Source: CAD feature listing. Evaluate the final solid. Frame: model axes, mm. A direction names the side the tool comes from. Round coordinates to 2 decimals unless told otherwise and drop trailing zeros. Order: outer loops, then holes, each group sorted by start corner. A loop starts at its lowest first (then second) coordinate and runs counter-clockwise, first axis right, second up. Notation, with made-up numbers: (67, 57) -> (100, 57) arc R18 cw to (100, 61) -> close; hole circle Ø3 at (52.25, 75.25). An arc over 180 degrees is marked (long way). One line per item, written item: value. Start each with the question number.
1) Section B-B (z = -34). Return the cut outline in (x, y) (1 decimal), and give its area (3 significant figures).
2) Mould query, pull axis X, two halves, no side actions, for faces 4 (the face through (12.7, 3, 28)), 5 (the face through (79, 3, -40.005)), 6 (the face through (16.43, 2.8, -14.05)), 7 (the face through (15.875, 3, 0)). Classes: pulls with the +X half, pulls with the -X half, needs draft (parallel to the pull), parting line crosses it, or undercut.
3) Section C-C (x = 33). Return the cut outline in (y, z) (3 decimals), and give its area (3 significant figures).
4) Section D-D (z = 5). Return the cut outline in (x, y) (1 decimal), and give its area (3 significant figures).
5) Pin query (flat end, axial travel): P1, Ø1.7, axis at y = 4, z = 11.5, coming from the +X side; P2, Ø3, axis at x = -7, y = 2, coming from the +Z side; P3, Ø1.6, axis at y = 3, z = -15, coming from the +X side. Return the tip coordinate at first contact, or that it passes through.
6) Section A-A (x = 0). Return the cut outline in (y, z) (3 decimals), and give its area (3 significant figures).
7) Reachability of faces 1 (the face through (74.295, 3, -36)), 2 (the face through (55.116, 2.885, -8.868)), 3 (the face through (28.499, 3, -32)) from +Z, -Z, +X, -X, +Y, -Y: full face, straight path, thin tool, end or side. Return the list, or none.
8) Ray query, L1, parallel to X at y = 5.05, z = -33 (1 decimal); L2, parallel to Z at x = 35, y = 3.15 (3 decimals); L3, parallel to X at y = 1.2, z = -26.67. Return the intervals inside material, ascending.
```python
from build123d import *

# Parameters (mm, degrees)
SKETCH1_W                   = 33.3375
SKETCH1_H                   = 41.1861
BOSS_EXTRUDE1_DEPTH         = 5.6896
FILLET1_R                   = 12.7
FILLET2_R                   = 6.35
CUT_EXTRUDE3_REACH          = 7.69
SKETCH11_R                  = 6.35
SKETCH8_W                   = 12.7
SKETCH8_H                   = 3.175
CUT_EXTRUDE2_DEPTH          = 5.6896
F_4_CLEARANCE_HOLE3_D       = 2.9464
F_4_CLEARANCE_HOLE3_DEPTH   = 5.6906
CIRPATTERN1_COUNT           = 4
FILLET3_R                   = 12.7
F_4_CLEARANCE_HOLE4_D       = 2.9464
TAP_DRILL_FOR_4_HELICOIL1_D = 3.9878
FILLET4_R                   = 6.35


with BuildPart() as part:
    # Sketch1 → Boss-Extrude1 (new body)
    with BuildSketch(Plane(origin=(0, 0, 0), x_dir=(1, 0, 0), z_dir=(0, 1, 0))):
        with BuildLine():
            Line((28.4988, 40.005), (28.4988, 24.13))
            Line((28.4988, 24.13), (0, 24.13))
            Line((0, 24.13), (-24.13, 24.13))
            Line((-24.13, 24.13), (-24.13, 0))
            Line((-24.13, 0), (-24.13, -24.13))
            Line((-24.13, -24.13), (0, -24.13))
            Line((0, -24.13), (12.7, -24.13))
            Line((12.7, -24.13), (12.7, -38.1))
            Line((12.7, -38.1), (71.8185, -38.1))
            Line((71.8185, -38.1), (71.8185, 7.9375))
            Line((71.8185, 7.9375), (84.5185, 20.6375))
            Line((84.5185, 20.6375), (84.5185, 40.005))
            Line((84.5185, 40.005), (74.295, 40.005))
            Line((74.295, 40.005), (74.295, 31.75))
            ThreePointArc((74.295, 31.75), (66.675, 24.13), (59.055, 31.75))
            Line((59.055, 31.75), (59.055, 40.005))
            Line((59.055, 40.005), (28.4988, 40.005))
        make_face()
        with Locations((42.06875, -7.90575)):
            Rectangle(SKETCH1_W, SKETCH1_H, mode=Mode.SUBTRACT)
    extrude(amount=BOSS_EXTRUDE1_DEPTH)

    # Fillet1
    fillet1_edges = [part.edges().sort_by_distance(p)[0] for p in [
        (58.7375, 2.8448, 28.4988),
        (58.7375, 2.8448, -12.6873),
    ]]
    fillet(fillet1_edges, radius=FILLET1_R)

    # Fillet2
    fillet2_edges = [part.edges().sort_by_distance(p)[0] for p in [
        (25.4, 2.8448, -12.6873),
        (25.4, 2.8448, 28.4988),
    ]]
    fillet(fillet2_edges, radius=FILLET2_R)

    # Sketch11 → Cut-Extrude3 (cut, up to next)
    with BuildSketch(Plane(origin=(0, 5.6896, 0), x_dir=(1, 0, 0), z_dir=(0, 1, 0)), mode=Mode.PRIVATE) as cut_extrude3_sk1:
        Circle(SKETCH11_R)
    cut_extrude3_tool1 = extrude(cut_extrude3_sk1.sketch, amount=-CUT_EXTRUDE3_REACH, mode=Mode.PRIVATE) & part.part
    add(cut_extrude3_tool1.solids().sort_by_distance((0, 5.6896, 0))[0], mode=Mode.SUBTRACT)

    # Sketch8 → Cut-Extrude2 (cut)
    with BuildSketch(Plane(origin=(0, 5.6896, 0), x_dir=(1, 0, 0), z_dir=(0, 1, 0))):
        with Locations((0, 14.2875)):
            Rectangle(SKETCH8_W, SKETCH8_H)
    cut_extrude2 = extrude(amount=-CUT_EXTRUDE2_DEPTH, mode=Mode.SUBTRACT)

    # #4 Clearance Hole3
    with Locations(Plane(origin=(0, 5.6896, 0), x_dir=(1, 0, 0), z_dir=(0, 1, 0))):
        with Locations((0, 9.525)):
            f_4_clearance_hole3 = Hole(F_4_CLEARANCE_HOLE3_D / 2, depth=F_4_CLEARANCE_HOLE3_DEPTH)

    # CirPattern1: Cut-Extrude2, #4 Clearance Hole3 ×4 about axis
    cirpattern1_axis = Axis((0, 0, 0), (0, 1, 0))
    for i in range(1, CIRPATTERN1_COUNT):
        add(cut_extrude2.rotate(cirpattern1_axis, i * 360 / CIRPATTERN1_COUNT), mode=Mode.SUBTRACT)
        add(f_4_clearance_hole3.rotate(cirpattern1_axis, i * 360 / CIRPATTERN1_COUNT), mode=Mode.SUBTRACT)

    # Fillet3
    fillet3_edges = [part.edges().sort_by_distance(p)[0] for p in [
        (71.8185, 2.8448, 38.1),
    ]]
    fillet(fillet3_edges, radius=FILLET3_R)

    # #4 Clearance Hole4 (through all)
    with Locations(Plane(origin=(0, 5.6896, 0), x_dir=(1, 0, 0), z_dir=(0, 1, 0))):
        with Locations((32.893, 36.83), (80.137, 36.83), (80.137, 26.67), (32.893, 26.67)):
            Hole(F_4_CLEARANCE_HOLE4_D / 2)

    # Tap Drill for #4 Helicoil1 (through all)
    with Locations(Plane(origin=(0, 5.6896, 0), x_dir=(1, 0, 0), z_dir=(0, 1, 0))):
        with Locations((-15.998290924, 15.998290924), (15.998290924, -15.998290924), (15.998290924, 15.998290924), (-15.998290924, -15.998290924), (0, 0)):
            Hole(TAP_DRILL_FOR_4_HELICOIL1_D / 2)

    # Fillet4
    fillet4_edges = [part.edges().sort_by_distance(p)[0] for p in [
        (12.7, 2.8448, 38.1),
        (-24.13, 2.8448, 24.13),
        (-24.13, 2.8448, -24.13),
    ]]
    fillet(fillet4_edges, radius=FILLET4_R)


solid = part.part
```
Findings:
1. outline: (28.5, 0) -> (59.1, 0) -> (59.1, 5.7) -> (28.5, 5.7) -> close; (74.3, 0) -> (84.5, 0) -> (84.5, 5.7) -> (74.3, 5.7) -> close
1. area: 232 mm2
2. face 4: pulls with the -X half
2. face 5: needs draft
2. face 6: undercut
2. face 7: undercut
3. outline: (0, -40.005) -> (5.69, -40.005) -> (5.69, -38.299) -> (0, -38.299) -> close; (0, -35.361) -> (5.69, -35.361) -> (5.69, -28.139) -> (0, -28.139) -> close; (0, -25.201) -> (5.69, -25.201) -> (5.69, -12.687) -> (0, -12.687) -> close; (0, 28.499) -> (5.69, 28.499) -> (5.69, 38.1) -> (0, 38.1) -> close
3. area: 177 mm2
4. outline: (-24.1, 0) -> (-15.9, 0) -> (-15.9, 5.7) -> (-24.1, 5.7) -> close; (-12.7, 0) -> (-3.9, 0) -> (-3.9, 5.7) -> (-12.7, 5.7) -> close; (3.9, 0) -> (12.7, 0) -> (12.7, 5.7) -> (3.9, 5.7) -> close; (15.9, 0) -> (25.4, 0) -> (25.4, 5.7) -> (15.9, 5.7) -> close; (58.7, 0) -> (71.8, 0) -> (71.8, 5.7) -> (58.7, 5.7) -> close
4. area: 276 mm2
5. P1: x = 71.82
5. P2: z = 24.13
5. P3: x = 79.68
6. outline: (0, -24.13) -> (5.69, -24.13) -> (5.69, -15.875) -> (0, -15.875) -> close; (0, -12.7) -> (5.69, -12.7) -> (5.69, -10.998) -> (0, -10.998) -> close; (0, -8.052) -> (5.69, -8.052) -> (5.69, -6.35) -> (0, -6.35) -> close; (0, 6.35) -> (5.69, 6.35) -> (5.69, 8.052) -> (0, 8.052) -> close; (0, 10.998) -> (5.69, 10.998) -> (5.69, 12.7) -> (0, 12.7) -> close; (0, 15.875) -> (5.69, 15.875) -> (5.69, 24.13) -> (0, 24.13) -> close
6. area: 133 mm2
7. face 1: -Z, +Y, -Y
7. face 2: +Y, -Y
7. face 3: -Z, -X, +Y, -Y
8. L1: 28.5 to 59.1, 74.3 to 84.5
8. L2: -40.005 to -12.687, 28.499 to 38.1
8. L3: 28.5 to 31.42, 34.37 to 61, 72.35 to 78.66, 81.61 to 84.52
